Source: CAD feature listing. Evaluate the final solid. Frame: model axes, mm. Face numbers are marked on the shaded views. Give positions to 0.01 mm unless a question says otherwise; leave off trailing zeros. Write each loop counter-clockwise with the first axis right and the second up, starting at its lowest first coordinate (ties: lowest second). Pieces come first, ordered by that corner, then holes. Notation, with made-up numbers: M 77,-28.5 L 121,-28.5 A22 cw 121,0.5 Z; hole C 78,-10 d1. An arc over 180 degrees is marked long. Use CSV: the item, a comma, the result in double quotes. Start each with the question number.
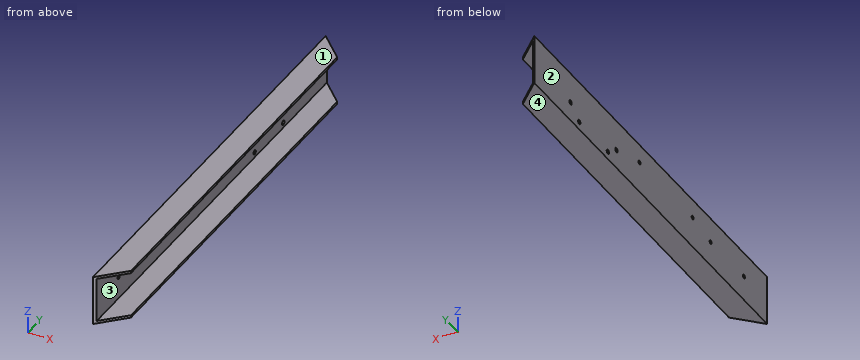
Solid Edge part; units mm, degrees
sketch "Sketch1" plane through (0, 0, 0) normal (0, -1, 0) x (1, 0, 0)
  line L0 (20, 36) -> (-16, 36)
  line L1 (-16, 36) -> (-16, -36)
  line L2 (-16, -36) -> (20, -36)
  line L3 (20, -36) -> (20, -40)
  line L4 (20, -40) -> (-20, -40)
  line L5 (-20, -40) -> (-20, 40)
  line L6 (-20, 40) -> (20, 40)
  line L7 (20, 40) -> (20, 36)
  dimension "D1" = 20
  dimension "D2" = 20
  dimension "D3" = 20
extrude "Protrusion1" add sketch "Sketch1" against normal blind 700
sketch "Sketch2" plane through (0, 350, 40) normal (0, 0, 1) x (0, 1, 0)
  line L0 (-350, 20) -> (-310, -20)
extrude "Cutout1" cut sketch "Sketch2" against normal through all material side at (0.0354, 19.9646, 40)
sketch "Sketch3" plane through (0, 350, 40) normal (0, 0, 1) x (0, 1, 0)
  line L0 (350, 20) -> (310, -20)
extrude "Cutout2" cut sketch "Sketch3" against normal through all material side at (0.0354, 680.0354, 40)
sketch "Sketch4" plane through (-16, 350, 0) normal (1, 0, 0) x (0, 1, 0)
  circle A0 centre (-126, 10) radius 3
  circle A1 centre (34, 10) radius 3
extrude "Cutout3" cut sketch "Sketch4" against normal through all
hole "Bohrung_1" at (-16, 591, -9.5) direction (-1, 0, 0) diameter 7 end up to next
hole "Hole1" at (-16, 565, -27.5) direction (-1, 0, 0) diameter 7 end up to next
hole "Hole2" at (-16, 453, -9.5) direction (-1, 0, 0) diameter 7 end up to next
hole "Hole3" at (-16, 479, -27.5) direction (-1, 0, 0) diameter 7 end up to next
sketch "Sketch5" plane through (-20, 350, 0) normal (-1, 0, 0) x (0, -1, 0)
  circle A0 centre (280, 0) radius 3
  circle A1 centre (180, 0) radius 3
  dimension "D1" = 280
  dimension "D2" = 280
extrude "Cutout4" cut sketch "Sketch5" against normal through all
properties part number "A1.1.M1" material "AlMgSi 0,5-1"
Item 1: Section B-B (y = 214). Return the cut outline in (x, z).
Item 2: Material intervals for probe 1 along Z at (x, y) = (-18.1, 591); probe 2 along Z at (x, y) = (6, 607.5); probe 3 along Y at (x, z) = (-18, -27), sorted ascending.
Item 3: Pull-direction query (Z, two-part tool) for the marked faces 1, 2, 3 and 4; classes: released by +Z, released by -Z, zero draft, split by the parting line, or undercut.
Item 4: Section A-A (x = 7). Return the cut outline in (y, z), plus the area to 3 significant figures.
Item 5: Section C-C (z = 25.5). Return the cut outline in (x, y), plus the area to 3 significant figures.
Item 6: Contact query for flat-ended pins moving along their axis: pin 1 Ø6 at (x, z) = (-15, 31.5) entering from +Y; pin 2 Ø2 at (y, z) = (210.5, 19) entering from +X; pin 3 Ø11 at (y, z) = (565, -27.5) entering from -X; pin 4 Ø3.5 at (y, z) = (224, 10) entering from -X. Output: stop coordinate, or through.
Output values:
1,outline,"M -20,-40 L 20,-40 L 20,-36 L -16,-36 L -16,36 L 20,36 L 20,40 L -20,40 Z"
2,probe 1,"z = -40 to -13, -6 to 40"
2,probe 2,"z = -40 to -36, 36 to 40"
2,probe 3,"y = 2 to 475.54, 482.46 to 561.54, 568.46 to 698"
3,face 1,"released by +Z"
3,face 2,"zero draft"
3,face 3,"undercut"
3,face 4,"released by -Z"
4,outline,"M 27,-40 L 673,-40 L 673,-36 L 27,-36 Z; M 27,36 L 673,36 L 673,40 L 27,40 Z"
4,area,"5,170 mm2"
5,outline,"M -20,0 L -16,4 L -16,696 L -20,700 Z"
5,area,"2,780 mm2"
6,pin 1,"stops at y = 698"
6,pin 2,"stops at x = -16"
6,pin 3,"stops at x = -20"
6,pin 4,"passes through"
